from build123d import *

# Parameters (mm, degrees)
SKETCH1_W           = 109.5
SKETCH1_H           = 90.5
SKETCH1_R           = 1.5
BOSS_EXTRUDE1_DEPTH = 1.5
SKETCH2_W           = 10
SKETCH2_H           = 15
BOSS_EXTRUDE2_DEPTH = 10
SKETCH3_W           = 14.7696301
SKETCH3_H           = 19.309368961
BOSS_EXTRUDE3_DEPTH = 2
SKETCH4_W           = 54.699442022
SKETCH4_H           = 29.942508018
BOSS_EXTRUDE4_DEPTH = 25
SKETCH5_W           = 9.03293538
SKETCH5_H           = 27.600635882
SKETCH5_W_2         = 7.52744615
SKETCH5_H_2         = 25.927870071
SKETCH5_W_3         = 22.080508706
SKETCH5_H_3         = 6.02195692
SKETCH5_W_4         = 8.97656987
SKETCH5_H_4         = 28.994339973
BOSS_EXTRUDE5_DEPTH = 10


with BuildPart() as part:
    # Sketch1 → Boss-Extrude1 (new body)
    with BuildSketch(Plane(origin=(0, 0, 0), x_dir=(1, 0, 0), z_dir=(0, 1, 0))):
        Rectangle(SKETCH1_W, SKETCH1_H)
        with Locations(Location((-52.45, -42.95, 0), (0, 0, 270))):
            Circle(SKETCH1_R, mode=Mode.SUBTRACT)
        with Locations(Location((-29.75, -12.45, 0), (0, 0, 270))):
            Circle(SKETCH1_R, mode=Mode.SUBTRACT)
        with Locations(Location((52.25, -42.95, 0), (0, 0, 270))):
            Circle(SKETCH1_R, mode=Mode.SUBTRACT)
        with Locations(Location((52.55, 43.05, 0), (0, 0, 270))):
            Circle(SKETCH1_R, mode=Mode.SUBTRACT)
        with Locations(Location((-51.75, 42.55, 0), (0, 0, 270))):
            Circle(SKETCH1_R, mode=Mode.SUBTRACT)
        with Locations(Location((-3.25, -7.45, 0), (0, 0, 270))):
            Circle(SKETCH1_R, mode=Mode.SUBTRACT)
        with Locations(Location((52.75, 15.75, 0), (0, 0, 270))):
            Circle(SKETCH1_R, mode=Mode.SUBTRACT)
    extrude(amount=BOSS_EXTRUDE1_DEPTH)

    # Sketch2 → Boss-Extrude2 (add)
    with BuildSketch(Plane(origin=(0, 1.5, 0), x_dir=(1, 0, 0), z_dir=(0, 1, 0))):
        with Locations((-39.75, -40.75)):
            Rectangle(SKETCH2_W, SKETCH2_H)
    extrude(amount=BOSS_EXTRUDE2_DEPTH)

    # Sketch3 → Boss-Extrude3 (add)
    with BuildSketch(Plane(origin=(0, 1.5, 0), x_dir=(1, 0, 0), z_dir=(0, 1, 0))):
        with Locations((-17.607300973, -39.57462345)):
            Rectangle(SKETCH3_W, SKETCH3_H)
    extrude(amount=BOSS_EXTRUDE3_DEPTH)

    # Sketch4 → Boss-Extrude4 (add)
    with BuildSketch(Plane(origin=(0, 1.5, 0), x_dir=(1, 0, 0), z_dir=(0, 1, 0))):
        with Locations((18.14950905, 20.509046194)):
            Rectangle(SKETCH4_W, SKETCH4_H)
    extrude(amount=BOSS_EXTRUDE4_DEPTH)

    # Sketch5 → Boss-Extrude5 (add)
    with BuildSketch(Plane(origin=(0, 1.5, 0), x_dir=(1, 0, 0), z_dir=(0, 1, 0))):
        with Locations((-47.004719291, -10.437121311)):
            Rectangle(SKETCH5_W, SKETCH5_H)
        with Locations((-46.251974676, 22.349088585)):
            Rectangle(SKETCH5_W_2, SKETCH5_H_2)
        with Locations((-27.935189045, 38.324002081)):
            Rectangle(SKETCH5_W_3, SKETCH5_H_3)
        with Locations((43.413693804, -27.937937952)):
            Rectangle(SKETCH5_W_4, SKETCH5_H_4)
    extrude(amount=BOSS_EXTRUDE5_DEPTH)


solid = part.part
Could you check a few things on this model? Use its own coordinates, in mm. A direction names the side the tool comes from. Coordinates: 2 decimals unless noted, no trailing zeros. Order: outer loops, then holes, each group sorted by start corner. A loop starts at its lowest first (then second) coordinate and runs counter-clockwise, first axis right, second up. Notation, with made-up numbers: (22.5, 13.5) -> (34.5, 13.5) arc R34 ccw to (34.5, 48.5) -> close; hole circle Ø3 at (8, 16). An arc over 180 degrees is marked (long way). One line per item, written item: value. Start each with the question number.
1) Imagine slicing it at D-D on x = 30.5. List the corners of the cut face in (y, z) for me, plus the area to 3 significant figures.
2) If I drill on L1, parallel to X at y = 1.25, z = 42.95; L2, parallel to X at y = 1.2, z = -15.75; L3, parallel to X at y = 24, z = -15, over which ranges is the centre line in solid material (lowest first)? Write a range as [from, to].
3) We'd pull the mould along Z, two halves only. Please class faces 1 (the flat face through (-46, 6, -35.313)), 2 (the flat face through (-38.975, 6, -38)), 3 (the cylindrical face through (-53.214, 0.74, -42.875)): +Z half, -Z half, draft (parallel to the pull), parting line (faces both ways), or undercut.
4) I'm going to push flat-ended pins straight in: pin 1 (3.5 mm diameter, centred on x = -51.75, z = -42.55, fed in from +Y); pin 2 (6 mm diameter, centred on y = 21, z = -21, fed in from +X); pin 3 (4 mm diameter, centred on x = -37.5, z = 37, fed in from +Y); pin 4 (2.5 mm diameter, centred on x = -52.45, z = 42.95, fed in from +Y). Where does each tip first touch, or does it pass through?
5) Imagine slicing it at B-B on y = 7.75. List the corners of the cut face in (x, z) for me, plus the area to 3 significant figures.
6) Imagine slicing it at C-C on z = 15.5. List the corners of the cut face in (x, y) for me, plus the area to 3 significant figures.
7) Imagine slicing it at A-A on x = -29.75. List the corners of the cut face in (y, z) for me.
8) Which directions (+Z, -Z, +X, -X, +Y, -Y) give clear straight access to the entire face, cutting with the end or side of a thin tool? Please do faces 4 (the flat face through (-40, 6, 33.25)), 5 (the flat face through (-42.488, 6, -22)), 6 (the flat face through (-18, 1.5, 47)), 7 (the flat face through (38.925, 6, 28)).
Answer list:
1. outline: (0, -45.25) -> (1.5, -45.25) -> (1.5, -35.48) -> (26.5, -35.48) -> (26.5, -5.54) -> (1.5, -5.54) -> (1.5, 45.25) -> (0, 45.25) -> close
1. area: 884 mm2
2. L1: x = [-54.75, -53.95], [-50.95, 50.75], [53.75, 54.75]
2. L2: x = [-54.75, 51.25], [54.25, 54.75]
2. L3: x = [-9.2, 45.5]
3. face 1: -Z half
3. face 2: draft
3. face 3: undercut
4. pin 1: stops at y = 1.5
4. pin 2: stops at x = 45.5
4. pin 3: stops at y = 11.5
4. pin 4: passes through
5. outline: (-51.52, -3.36) -> (-42.49, -3.36) -> (-42.49, 24.24) -> (-51.52, 24.24) -> close; (-50.02, -35.31) -> (-42.49, -35.31) -> (-42.49, -9.39) -> (-50.02, -9.39) -> close; (-44.75, 33.25) -> (-34.75, 33.25) -> (-34.75, 48.25) -> (-44.75, 48.25) -> close; (-38.98, -41.33) -> (-16.89, -41.33) -> (-16.89, -35.31) -> (-38.98, -35.31) -> close; (-9.2, -35.48) -> (45.5, -35.48) -> (45.5, -5.54) -> (-9.2, -5.54) -> close; (38.93, 13.44) -> (47.9, 13.44) -> (47.9, 42.44) -> (38.93, 42.44) -> close
5. area: 2,630 mm2
6. outline: (-54.75, 0) -> (54.75, 0) -> (54.75, 1.5) -> (47.9, 1.5) -> (47.9, 11.5) -> (38.93, 11.5) -> (38.93, 1.5) -> (-42.49, 1.5) -> (-42.49, 11.5) -> (-51.52, 11.5) -> (-51.52, 1.5) -> (-54.75, 1.5) -> close
6. area: 344 mm2
7. outline: (0, -45.25) -> (1.5, -45.25) -> (1.5, -41.33) -> (11.5, -41.33) -> (11.5, -35.31) -> (1.5, -35.31) -> (1.5, 10.95) -> (0, 10.95) -> close; (0, 13.95) -> (1.5, 13.95) -> (1.5, 45.25) -> (0, 45.25) -> close
8. face 4: -X, +Y
8. face 5: -Z, +Y
8. face 6: +Z, +X, -X, -Y
8. face 7: +Z, +Y
